```python
from build123d import *

# Parameters (mm, degrees)
BOSS_EXTRUDE1_DEPTH     = 40
SHELL1_T                = -2
SKETCH2_W               = 1.5
SKETCH2_H               = 6.3
SKETCH2_W_2             = 2.058506146
SKETCH2_H_2             = 3.660298136
CUT_EXTRUDE1_DEPTH      = 25
SKETCH3_W               = 1
SKETCH3_H               = 15
CUT_EXTRUDE2_DEPTH      = 1
CUT_EXTRUDE2_DEPTH_BACK = 31


with BuildPart() as part:
    # Sketch1 → Boss-Extrude1 (new body)
    with BuildSketch(Plane.XY):
        with BuildLine():
            Line((-7.5, -20), (7.5, -20))
            ThreePointArc((7.5, -20), (12.803300859, -17.803300859), (15, -12.5))
            Line((15, -12.5), (15, 12.5))
            ThreePointArc((15, 12.5), (12.803300859, 17.803300859), (7.5, 20))
            Line((7.5, 20), (-7.5, 20))
            ThreePointArc((-7.5, 20), (-12.803300859, 17.803300859), (-15, 12.5))
            Line((-15, 12.5), (-15, -12.5))
            ThreePointArc((-15, -12.5), (-12.803300859, -17.803300859), (-7.5, -20))
        make_face()
    extrude(amount=BOSS_EXTRUDE1_DEPTH)

    # Shell1
    shell1_openings = [part.faces().sort_by_distance(p)[0] for p in [
        (0, 0, 40),
    ]]
    offset(amount=SHELL1_T, openings=shell1_openings, kind=Kind.INTERSECTION)

    # Sketch2 → Cut-Extrude1 (cut)
    with BuildSketch(Plane(origin=(0, 0, 0), x_dir=(-1, 0, 0), z_dir=(0, 0, -1))):
        with Locations((-5.6, 4.85)):
            Rectangle(SKETCH2_W, SKETCH2_H)
        with Locations((7.1, 4.85)):
            Rectangle(SKETCH2_W, SKETCH2_H)
        with Locations((0.75, -7.05)):
            Rectangle(SKETCH2_W_2, SKETCH2_H_2)
    extrude(amount=-CUT_EXTRUDE1_DEPTH, mode=Mode.SUBTRACT)

    # Sketch3 → Cut-Extrude2 (cut, two sides)
    with BuildSketch(Plane.ZY.offset(15)) as cut_extrude2_sk:
        with Locations((8.174979933, 1.491514735)):
            Rectangle(SKETCH3_W, SKETCH3_H)
        with Locations((6.174979933, 1.491514735)):
            Rectangle(SKETCH3_W, SKETCH3_H)
        with Locations((10.174979933, 1.491514735)):
            Rectangle(SKETCH3_W, SKETCH3_H)
        with Locations((12.174979933, 1.491514735)):
            Rectangle(SKETCH3_W, SKETCH3_H)
        with Locations((14.174979933, 1.491514735)):
            Rectangle(SKETCH3_W, SKETCH3_H)
    extrude(amount=CUT_EXTRUDE2_DEPTH, mode=Mode.SUBTRACT)
    extrude(cut_extrude2_sk.sketch, amount=-CUT_EXTRUDE2_DEPTH_BACK, mode=Mode.SUBTRACT)


solid = part.part
```
The model under review builds one solid part; all positions refer to its coordinate system, in mm. A direction names the side the tool comes from. Round coordinates to 2 decimals unless told otherwise and drop trailing zeros. Loops run counter-clockwise (first coordinate to the right, second up) from the corner with the lowest first, then second, coordinate; pieces in that order, holes last.
1) Consider section A-A on z = 21. State the section outline as (x, y) points, then the cut area to 3 significant figures.
Values follow:
outline: (-15, -12.5) arc R7.5 ccw to (-7.5, -20) - (7.5, -20) arc R7.5 ccw to (15, -12.5) - (15, 12.5) arc R7.5 ccw to (7.5, 20) - (-7.5, 20) arc R7.5 ccw to (-15, 12.5) - close; hole (-13, -12.5) arc R5.5 ccw to (-7.5, -18) - (7.5, -18) arc R5.5 ccw to (13, -12.5) - (13, 12.5) arc R5.5 ccw to (7.5, 18) - (-7.5, 18) arc R5.5 ccw to (-13, 12.5) - close
area: 242 mm2
2) Consider section B-B on y = -8. State the section outline as (x, z) points.
Values follow:
outline: (-15, 0) - (-1.78, 0) - (-1.78, 2) - (-13, 2) - (-13, 40) - (-15, 40) - close; (0.28, 0) - (15, 0) - (15, 40) - (13, 40) - (13, 2) - (0.28, 2) - close
3) The part is to be moulded in two halves that separate along Z. For faces 4 (the face through (-14, -6.008, 10)), 5 (the face through (0, 0, 2)), 6 (the face through (-6.35, 5, 1)), say which applies: pulls with the +Z half, pulls with the -Z half, needs draft (parallel to the pull), parting line crosses it, or undercut.
Values follow:
face 4: undercut
face 5: pulls with the +Z half
face 6: needs draft
4) Clearance check with flat-ended pins moving along their axes: P1, Ø0.5, axis at x = 13.5, z = 8, coming from the +Y side; P2, Ø0.5, axis at x = 14, z = 14.5, coming from the -Y side; P3, Ø0.5, axis at x = 14, z = 10, coming from the +Y side. State where each tip first meets the part, or that it passes through.
Values follow:
P1: stops at y = 17.32
P2: stops at y = -16.65
P3: stops at y = 16.65
5) Wall thickness on line 1 along X through (y, z) = (10.5, 35.5); line 2 along Y through (x, z) = (0.25, 4.5); line 3 along Z through (x, y) = (6.5, 8): over which ranges is each line inside the solid? List them lowest first.
Values follow:
line 1: x = -15 to -13, 13 to 15
line 2: y = -20 to -18, 18 to 20
line 3: z = 0 to 2
6) Tool access review of faces 1 (the face through (4.85, 5, 1)), 2 (the face through (14, 8.992, 14)), 3 (the face through (13, 0, 21)): name each direction out of +Z, -Z, +X, -X, +Y, -Y from which nothing blocks a thin tool from reaching the whole face with its end or side.
Values follow:
face 1: +Z, -Z
face 2: +X, -X
face 3: +Z
7) Consider section D-D on y = 5. Give the number of separate pieces and of enclosed holes in the cut face, then the cut area to 3 significant figures.
Values follow:
separate pieces: 13
enclosed holes: 0
area: 186 mm2
8) Consider section C-C on x = -11.5. State the section outline as (y, z) points, then the cut area to 3 significant figures.
Values follow:
outline: (-18.84, 0) - (18.84, 0) - (18.84, 40) - (16.27, 40) - (16.27, 2) - (-16.27, 2) - (-16.27, 40) - (-18.84, 40) - close
area: 271 mm2
